CAD build for the part. Positions are in the model's coordinates, mm. A direction names the side the tool comes from. Coordinates: 2 decimals unless noted, no trailing zeros. Loops run counter-clockwise (first coordinate to the right, second up) from the corner with the lowest first, then second, coordinate; pieces in that order, holes last. Notation, with made-up numbers: (-1.5, -15) -> (40.5, -15) arc R11 cw to (40.5, -2) -> close; hole circle Ø5 at (24.25, 22). An arc over 180 degrees is marked (long way). Answer as CSV lines item,"result". Start each with the question number.
from build123d import *

# Parameters (mm, degrees)
F0_R     = 7.9375
F0_R_2   = 6.35
F1_DEPTH = 2.032
F4_DEPTH = 1.27
F5_R     = 2.54
F6_R     = 0.635


with BuildPart() as f1:
    # F0 (on Top) → F1 (new body)
    with BuildSketch(Plane.XY):
        Circle(F0_R)
        Circle(F0_R_2, mode=Mode.SUBTRACT)
    extrude(amount=F1_DEPTH)

    # F3 (on offset) → F4 (join, symmetric)
    with BuildSketch(Plane.YZ.offset(7.874)):
        Polygon((-6.665544, 0), (7.295991, 0), (7.934471, 8.52365), (1.720515, 8.52365), (2.570548, 3.045656), (-5.269391, 3.045656), (-8.920868, 6.589739), (-8.920868, 4.119621), align=None)
    extrude(amount=F4_DEPTH, both=True)

    # F5
    f5_edges = [f1.edges().sort_by_distance(p)[0] for p in [
        (7.874, 2.570548, 3.045656),
        (7.874, -5.269391, 3.045656),
        (7.874, 7.295991, 0),
        (7.874, -6.665544, 0),
        (7.874, -8.920868, 4.119621),
    ]]
    fillet(f5_edges, radius=F5_R)

    # F6
    f6_edges = [f1.edges().sort_by_distance(p)[0] for p in [
        (7.874, -8.920868, 6.589739),
    ]]
    fillet(f6_edges, radius=F6_R)


solid = f1.part
Item 1: Two-plate mould, pull along Y, no slides. Class faces 1 (the face through (6, 3, 0)), 2 (the face through (7.86, -8.54, 5.67)), 3 (the face through (7.89, 6.65, 0.66)): pulls with the +Y half, pulls with the -Y half, needs draft (parallel to the pull), parting line crosses it, or undercut.
Item 2: Wall check: probe 1 along Y at (x, z) = (-0.25, 1); probe 2 along X at (y, z) = (5.5, 1.25); probe 3 along Z at (x, y) = (-4.5, 6.25). Give the ranges that are in metal, low to high.
Item 3: Which spindle directions (+Z, -Z, +X, -X, +Y, -Y) get a long thin tool onto all of the face, cutting with end or side? Do faces 4 (the face through (7.892, 1.555, 3.956)), 5 (the face through (7.856, -6.439, 0.345)), 6 (the face through (8, -2, 3.046)), 7 (the face through (-6.1, 2.4, 2.032)). Say none if no direction does.
Item 4: Saw through at A-A (x = 0). Write the cut outline in (y, z), plus the area to 3 significant figures.
Item 5: Flat gauge pins, fed straight in: pin 1 Ø2 at (x, y) = (8.5, -2.5) entering from +Z; pin 2 Ø5 at (y, z) = (-2.5, 5) entering from -X; pin 3 Ø1.5 at (x, z) = (-1.5, 4.5) entering from +Y. Where does each tip first touch, or does it go through?
Item 6: Saw through at B-B (y = -1). Write the cut outline in (x, z), plus the area to 3 significant figures.
Geometry check:
1,face 1,"needs draft"
1,face 2,"undercut"
1,face 3,"pulls with the +Y half"
2,probe 1,"-7.93 to -6.35, 6.35 to 7.93"
2,probe 2,"-5.72 to -3.17, 3.17 to 5.72, 6.6 to 9.14"
2,probe 3,"0 to 2.03"
3,face 4,"+X, -X"
3,face 5,"-Z, +X, -Y"
3,face 6,"+Z, +X, -X"
3,face 7,"+Z, -X, +Y, -Y"
4,outline,"(-7.94, 0) -> (-6.35, 0) -> (-6.35, 2.03) -> (-7.94, 2.03) -> close; (6.35, 0) -> (7.94, 0) -> (7.94, 2.03) -> (6.35, 2.03) -> close"
4,area,"6.45 mm2"
5,pin 1,"z = 3.05"
5,pin 2,"x = 6.6"
5,pin 3,"through"
6,outline,"(-7.87, 0) -> (-6.27, 0) -> (-6.27, 2.03) -> (-7.87, 2.03) -> close; (6.27, 0) -> (9.14, 0) -> (9.14, 3.05) -> (6.6, 3.05) -> (6.6, 2.03) -> (6.27, 2.03) -> close"
6,area,"11.7 mm2"
